from build123d import *

# Parameters (mm, degrees)
BOSS_EXTRUDE1_DEPTH = 304.8
SKETCH2_W           = 25.4
SKETCH2_H           = 6.35
BOSS_EXTRUDE2_DEPTH = 6.35
LPATTERN1_COUNT     = 6
LPATTERN1_PITCH     = 50.8
SKETCH3_R           = 1.25
CUT_EXTRUDE1_DEPTH  = 6.35
BOSS_EXTRUDE3_DEPTH = 6.35
LPATTERN2_COUNT     = 2
LPATTERN2_PITCH     = 38.1
CUT_EXTRUDE2_DEPTH  = 319.521766414
CUT_EXTRUDE3_DEPTH  = 319.521766414
SKETCH7_R           = 2.0955
CUT_EXTRUDE4_DEPTH  = 319.521766414
SKETCH8_W           = 31.75
SKETCH8_H           = 63.5
CUT_EXTRUDE5_DEPTH  = 319.521766414
FILLET1_R           = 3.81


with BuildPart() as part:
    # Sketch1 → Boss-Extrude1 (new body)
    with BuildSketch(Plane.XY):
        Polygon((37.717075708, 7.683880312), (33.226947648, 12.174008373), (69.147972132, 48.095032857), (73.638100193, 43.604904797), align=None)
    extrude(amount=BOSS_EXTRUDE1_DEPTH)

    # Sketch2 → Boss-Extrude2 (add)
    with BuildSketch(Plane(origin=(58.621502495, 58.621502495, 0), x_dir=(0, 0, -1), z_dir=(0.7071067811865471, 0.7071067811865479, 0))):
        with Locations((-266.7, -18.061676125)):
            Rectangle(SKETCH2_W, SKETCH2_H)
    boss_extrude2 = extrude(amount=BOSS_EXTRUDE2_DEPTH)

    # LPattern1: Boss-Extrude2 ×6
    with Locations(*[(0, 0, -i * LPATTERN1_PITCH) for i in range(1, LPATTERN1_COUNT)]):
        add(boss_extrude2)

    # Sketch3 → Cut-Extrude1 (cut)
    with BuildSketch(Plane(origin=(15.016597698, -15.016597698, 0), x_dir=(0, 0, -1), z_dir=(0.7071067811865396, -0.7071067811865555, 0))):
        with Locations(Location((-273.3375, 57.503323875, 0), (0, 0, 90))):
            Circle(SKETCH3_R)
    extrude(amount=-CUT_EXTRUDE1_DEPTH, mode=Mode.SUBTRACT)

    # Sketch4 → Boss-Extrude3 (add)
    with BuildSketch(Plane(origin=(0, 0, 0), x_dir=(-1, 0, 0), z_dir=(0, 0, -1))):
        Polygon((-33.226947648, 12.174008373), (-37.717075708, 7.683880312), (-46.69733183, 16.664136433), (-42.207203769, 21.154264494), align=None)
    boss_extrude3 = extrude(amount=BOSS_EXTRUDE3_DEPTH)

    # LPattern2: Boss-Extrude3 ×2
    with Locations(*[Vector(0.7071067811865472, 0.7071067811865478, 0) * (i * LPATTERN2_PITCH) for i in range(1, LPATTERN2_COUNT)]):
        add(boss_extrude3)

    # Sketch5 → Cut-Extrude2 (cut, through all)
    with BuildSketch(Plane(origin=(10.526469638, -10.526469638, 0), x_dir=(0.7071067811865537, 0.7071067811865415, 0), z_dir=(-0.7071067811865415, 0.7071067811865537, 0))):
        Polygon((59.636923875, 0), (55.369723875, 0), (55.369723875, -8.763), (53.058323875, -8.763), (53.058323875, -11.938), (55.369723875, -11.938), (55.369723875, -15.24), (59.636923875, -15.24), (59.636923875, -11.938), (61.948323875, -11.938), (61.948323875, -8.763), (59.636923875, -8.763), align=None)
    extrude(amount=-CUT_EXTRUDE2_DEPTH, mode=Mode.SUBTRACT)

    # Sketch6 → Cut-Extrude3 (cut, through all)
    with BuildSketch(Plane(origin=(10.526469638, -10.526469638, 0), x_dir=(0.7071067811865537, 0.7071067811865415, 0), z_dir=(-0.7071067811865415, 0.7071067811865537, 0))):
        Polygon((82.903323875, -294.2336), (82.903323875, -289.9664), (74.140323875, -289.9664), (74.140323875, -287.655), (70.965323875, -287.655), (70.965323875, -289.9664), (67.663323875, -289.9664), (67.663323875, -294.2336), (70.965323875, -294.2336), (70.965323875, -296.545), (74.140323875, -296.545), (74.140323875, -294.2336), align=None)
        Polygon((82.903323875, -40.2336), (82.903323875, -35.9664), (74.140323875, -35.9664), (74.140323875, -33.655), (70.965323875, -33.655), (70.965323875, -35.9664), (67.663323875, -35.9664), (67.663323875, -40.2336), (70.965323875, -40.2336), (70.965323875, -42.545), (74.140323875, -42.545), (74.140323875, -40.2336), align=None)
    extrude(amount=-CUT_EXTRUDE3_DEPTH, mode=Mode.SUBTRACT)

    # Sketch7 → Cut-Extrude4 (cut, through all)
    with BuildSketch(Plane(origin=(15.016597698, -15.016597698, 0), x_dir=(-0.7071067811865553, -0.7071067811865398, 0), z_dir=(0.7071067811865398, -0.7071067811865553, 0))):
        with Locations(Location((-86.078323875, -215.828690193, 0), (0, 0, 180))):
            Circle(SKETCH7_R)
        with Locations(Location((-86.078323875, -63.428690193, 0), (0, 0, 180))):
            Circle(SKETCH7_R)
    extrude(amount=-CUT_EXTRUDE4_DEPTH, mode=Mode.SUBTRACT)

    # Sketch8 → Cut-Extrude5 (cut, through all)
    with BuildSketch(Plane(origin=(10.526469638, -10.526469638, 0), x_dir=(0.7071067811865537, 0.7071067811865415, 0), z_dir=(-0.7071067811865415, 0.7071067811865537, 0))):
        with Locations((47.978323875, -165.1)):
            Rectangle(SKETCH8_W, SKETCH8_H)
    extrude(amount=-CUT_EXTRUDE5_DEPTH, mode=Mode.SUBTRACT)

    # Fillet1
    fillet1_edges = [part.edges().sort_by_distance(p)[0] for p in [
        (35.472011678, 9.928944343, 196.85),
        (35.472011678, 9.928944343, 133.35),
        (57.922651981, 32.379584645, 133.35),
        (57.922651981, 32.379584645, 196.85),
    ]]
    fillet(fillet1_edges, radius=FILLET1_R)


solid = part.part
Check sheet for the modelled part. Datum: model origin and axes. Units: mm. A direction names the side the tool comes from. Coordinates: 2 decimals unless noted, no trailing zeros. Write each loop counter-clockwise with the first axis right and the second up, starting at its lowest first coordinate (ties: lowest second). Pieces come first, ordered by that corner, then holes.
Item 1: Cross-section at B-B on z = 188.5. Record the boundary of the cut face in (x, y).
Numbers:
outline: (55.68, 34.62) - (60.17, 30.13) - (73.64, 43.6) - (69.15, 48.1) - close
Item 2: Depth check by flat-ended pin: pin 1 Ø3 at (y, z) = (28, 100) entering from +X; pin 2 Ø1 at (y, z) = (31, 108.5) entering from +X; pin 3 Ø3 at (x, z) = (52, 33) entering from -Y; pin 4 Ø10 at (x, y) = (73.5, 47.5) entering from -Z. Enter the tip coordinate at first touch or a pass-through.
Numbers:
pin 1: stops at x = 59.53
pin 2: stops at x = 61.53
pin 3: stops at y = 20.47
pin 4: stops at z = -6.35
Item 3: Cross-section at A-A on z = 156.5. Record the boundary of the cut face in (x, y), then the cut area to 3 significant figures.
Numbers:
outline: (55.68, 34.62) - (60.17, 30.13) - (78.13, 48.1) - (73.64, 52.59) - close
area: 161 mm2
Item 4: Mould release check, pull along Z, two halves, no side actions. Record for faces 1 (the face through (51, 26, 11.938)), 2 (the face through (74, 48, 101.6)), 3 (the face through (54, 28, 304.8)), 4 (the face through (67, 41, -6.35)): released by +Z, released by -Z, zero draft, split by the parting line, or undercut.
Numbers:
face 1: undercut
face 2: undercut
face 3: released by +Z
face 4: released by -Z
Item 5: Access from +Z, -Z, +X, -X, +Y, -Y to the whole of each face (thin tool, end or side, straight path). Record for faces 5 (the face through (74, 48, 25.4)), 6 (the face through (64, 39, 296.545)), 7 (the face through (36.272, 10.666, 197.996)), 8 (the face through (68, 43, 294.234)).
Numbers:
face 5: +X, +Y
face 6: none
face 7: -X, -Y
face 8: +X, -X, +Y, -Y
Item 6: Scan lines: probe 1 along Z at (x, y) = (46, 21.5); probe 2 along Z at (x, y) = (59.5, 30.5); probe 3 along Y at (x, z) = (44, 229.5). Record each from-to range of solid material in increasing order.
Numbers:
probe 1: z = 0 to 133.35, 196.85 to 304.8
probe 2: z = 0 to 135.9, 194.3 to 304.8
probe 3: y = 13.97 to 22.95
